Geometry check sheet. Reference: the model listing, model coordinates, mm. A direction names the side the tool comes from. Coordinates: 2 decimals unless noted, no trailing zeros. Order: outer loops, then holes, each group sorted by start corner. A loop starts at its lowest first (then second) coordinate and runs counter-clockwise, first axis right, second up. Notation, with made-up numbers: (58, 15.25) - (92, 15.25) arc R36 ccw to (92, 54.25) - close; hole circle Ø6 at (-18, 74.5). An arc over 180 degrees is marked (long way). Return JSON: item names as keys, results as strings. Group by question number.
Item 1: Section check C-C on x = 6.5. Enter the section's corners in (y, z), then the cut area to 3 significant figures.
Item 2: Draft check along Y on faces 1 (the flat face through (-11, 34, 6)), 2 (the flat face through (-32, 21, 16)), 3 (the flat face through (36, -8, 14.999)). Enter one of: pulls with the +Y half, pulls with the -Y half, needs draft (parallel to the pull), parting line crosses it, or undercut.
Item 3: Tool access check on faces 4 (the flat face through (-3, 46, 3)), 5 (the flat face through (0, 12, 10)), 6 (the flat face through (33, 34, 6)). Record the directions out of +Z, -Z, +X, -X, +Y, -Y that give a thin tool (end or side, any length) a straight path to the whole face; none if there is none.
Item 4: Scan lines: probe 1 along X at (y, z) = (42.5, 17); probe 2 along Y at (x, z) = (-20.5, 6.5); probe 3 along Y at (x, z) = (-4, 7.5). Record each from-to range of solid material in increasing order.
Item 5: Gauge pin test, flat ends, axial feed: pin 1 (6 mm diameter, centred on x = 28, z = 20.5, fed in from +Y); pin 2 (5 mm diameter, centred on x = -37, y = -11.5, fed in from +Z); pin 3 (8 mm diameter, centred on x = 12, y = -8.5, fed in from -Z). Record the tip position at first contact, or that the pin passes through.
Item 6: Section check A-A on y = 30.5. Enter the section's corners in (x, z), then the cut area to 3 significant figures.
Item 7: Section check D-D on z = 3. Enter the section's corners in (x, y), then the cut area to 3 significant figures.
Item 8: Section check B-B on z = 13. Enter the section's corners in (x, y), then the cut area to 3 significant figures.
from build123d import *

# Parameters (mm, degrees)
EXTRUDE_1_DEPTH     = 26
SKETCH_3_W          = 40
SKETCH_3_H          = 36
CUT_EXTRUDE_4_DEPTH = 20
SKETCH_4_W          = 20
SKETCH_4_H          = 20
CUT_EXTRUDE_5_DEPTH = 25
CUT_EXTRUDE_3_DEPTH = 8
CUT_EXTRUDE_6_DEPTH = 8
CUT_EXTRUDE_7_DEPTH = 16
CUT_EXTRUDE_8_DEPTH = 16


with BuildPart() as part:
    # 草图1 → 凸台-拉伸1 (new body)
    with BuildSketch(Plane.XY):
        Polygon((-34, -24), (34, -24), (44, 23), (44, 46), (-44, 46), (-44, 23), align=None)
    extrude(amount=EXTRUDE_1_DEPTH)

    # 草图3 → 切除-拉伸4 (cut)
    with BuildSketch(Plane(origin=(0, 0, 0), x_dir=(-1, 0, 0), z_dir=(0, 0, -1))):
        with Locations((0, -6)):
            Rectangle(SKETCH_3_W, SKETCH_3_H)
    extrude(amount=-CUT_EXTRUDE_4_DEPTH, mode=Mode.SUBTRACT)

    # 草图4 → 切除-拉伸5 (cut)
    with BuildSketch(Plane(origin=(0, 46, 0), x_dir=(1, 0, 0), z_dir=(0, 1, 0))):
        with Locations((33, -16)):
            Rectangle(SKETCH_4_W, SKETCH_4_H)
        with Locations((11, -16)):
            Rectangle(SKETCH_4_W, SKETCH_4_H)
        with Locations((-11, -16)):
            Rectangle(SKETCH_4_W, SKETCH_4_H)
        with Locations((-32, -16)):
            Rectangle(SKETCH_4_W, SKETCH_4_H)
    extrude(amount=-CUT_EXTRUDE_5_DEPTH, mode=Mode.SUBTRACT)

    # Sketch 3D_5 → 切除-拉伸3 (cut, symmetric)
    with BuildSketch(Plane(origin=(-26.633413551, -5.666683734, 23.004025099), x_dir=(-0.691625335103945, -0.14715432661786076, 0.7071067811865475), z_dir=(-0.2081076444648591, 0.9781059289848354, 0))):
        with BuildLine():
            Line((0, 0), (5.656854249, 5.656854249))
            Line((5.656854249, 5.656854249), (11.313708499, 0))
            ThreePointArc((11.313708499, 0), (5.656854249, -13.656854249), (0, 0))
        make_face()
    extrude(amount=CUT_EXTRUDE_3_DEPTH, both=True, mode=Mode.SUBTRACT)

    # Sketch 3D_6 → 切除-拉伸6 (cut, symmetric)
    with BuildSketch(Plane(origin=(34.478414998, -7.335832978, 14.99907516), x_dir=(0.5895982688198705, -0.12544644017993214, 0.7978954016979886), z_dir=(-0.20810764446495697, -0.9781059289848145, -6.6559639472978385e-12))):
        with BuildLine():
            Line((0, 0), (6.376045072, -8.439700449))
            Line((6.376045072, -8.439700449), (17.547318622, 0))
            Line((17.547318622, 0), (11.17127355, 8.439700449))
            Line((11.17127355, 8.439700449), (6.348906145, 14.822863662))
            Line((6.348906145, 14.822863662), (1.560795809, 11.205530619))
            ThreePointArc((1.560795809, 11.205530619), (-1.540343474, 5.926016705), (0, 0))
        make_face()
    extrude(amount=CUT_EXTRUDE_6_DEPTH, both=True, mode=Mode.SUBTRACT)

    # 草图7 → 切除-拉伸7 (cut)
    with BuildSketch(Plane(origin=(-1.664861156, 7.824847432, 0), x_dir=(0.9781059289848355, 0.2081076444648587, 0), z_dir=(0.2081076444648587, -0.9781059289848355, 0))):
        with BuildLine():
            Line((-24.556702047, 20), (-31.200844281, 16.10051891))
            ThreePointArc((-31.200844281, 16.10051891), (-33.152072653, 15.280030806), (-35.250185053, 15))
            Line((-35.250185053, 15), (-43.250185053, 15))
            Line((-43.250185053, 15), (-43.250185053, 23))
            ThreePointArc((-43.250185053, 23), (-40.3181561, 29.189965223), (-33.671267687, 30.842641134))
            Line((-33.671267687, 30.842641134), (-10.087245225, 28.492198282))
            Line((-10.087245225, 28.492198282), (-24.556702047, 20))
        make_face()
    extrude(amount=CUT_EXTRUDE_7_DEPTH, mode=Mode.SUBTRACT)

    # 草图11 → 切除-拉伸8 (cut)
    with BuildSketch(Plane(origin=(-1.664861156, -7.824847432, 0), x_dir=(0.9781059289845859, -0.2081076444660318, -1.1269708570671002e-12), z_dir=(0.20810764446603178, 0.9781059289845858, 5.296763028184159e-12))):
        with BuildLine():
            Line((31.200844283, -16.100518909), (14.333584528, -26))
            Line((14.333584528, -26), (32.666556858, -30.571318601))
            ThreePointArc((32.666556858, -30.571318601), (42.196349228, -26.968728166), (40.460809076, -16.92962956))
            Line((40.460809076, -16.92962956), (38.250185053, -14.99907516))
            Line((38.250185053, -14.99907516), (35.250185053, -15))
            ThreePointArc((35.250185053, -15), (33.152072655, -15.280030806), (31.200844283, -16.100518909))
        make_face()
    extrude(amount=CUT_EXTRUDE_8_DEPTH, mode=Mode.SUBTRACT)


solid = part.part
Computed:
{
 "1": {"outline": "(-24, 20) - (12, 20) - (12, 0) - (46, 0) - (46, 6) - (21, 6) - (21, 26) - (-24, 26) - close", "area": "600 mm²"},
 "2": {"face 1": "needs draft", "face 2": "pulls with the +Y half", "face 3": "undercut"},
 "3": {"face 4": "+Z, -Z, +X, -X, +Y", "face 5": "-Z, -Y", "face 6": "+Z, +Y"},
 "4": {"probe 1": "x = -44 to -42, -22 to -21, -1 to 1, 21 to 23, 43 to 44", "probe 2": "y = -24 to 21", "probe 3": "y = 12 to 21"},
 "5": {"pin 1": "stops at y = 21", "pin 2": "stops at z = 15", "pin 3": "stops at z = 20"},
 "6": {"outline": "(-44, 0) - (44, 0) - (44, 26) - (43, 26) - (43, 6) - (23, 6) - (23, 26) - (21, 26) - (21, 6) - (1, 6) - (1, 26) - (-1, 26) - (-1, 6) - (-21, 6) - (-21, 26) - (-22, 26) - (-22, 6) - (-42, 6) - (-42, 26) - (-44, 26) - close", "area": "688 mm²"},
 "7": {"outline": "(-44, 23) - (-34, -24) - (-20, -24) - (-20, 12) - (20, 12) - (20, -24) - (34, -24) - (44, 23) - (44, 46) - (-44, 46) - close", "area": "4,250 mm²"},
 "8": {"outline": "(-44, 23) - (-34, -24) - (-20, -24) - (-20, 12) - (20, 12) - (20, -24) - (34, -24) - (44, 23) - (44, 46) - (43, 46) - (43, 21) - (23, 21) - (23, 46) - (21, 46) - (21, 21) - (1, 21) - (1, 46) - (-1, 46) - (-1, 21) - (-21, 21) - (-21, 46) - (-22, 46) - (-22, 21) - (-42, 21) - (-42, 46) - (-44, 46) - close", "area": "2,250 mm²"}
}
